Read the model definition and answer for the solid it produces. Units are mm, in the model's axes. Face numbers are marked on the shaded views. Give positions to 0.01 mm unless a question says otherwise; leave off trailing zeros. Order: outer loops, then holes, each group sorted by start corner. A loop starts at its lowest first (then second) coordinate and runs counter-clockwise, first axis right, second up. Notation, with made-up numbers: M -7.75,74.5 L 35.25,74.5 A33 ccw 35.25,106.5 Z; hole C 51.25,34.5 d9. An arc over 180 degrees is marked long. One line per item, written item: value.
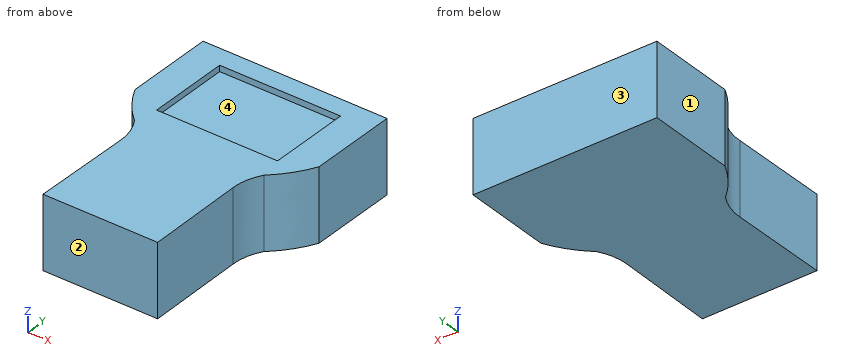
from build123d import *

# Parameters (mm, degrees)
BOSS_EXTRUDE1_DEPTH = 30
SKETCH2_W           = 50.095183997
SKETCH2_H           = 33.986838613
CUT_EXTRUDE1_DEPTH  = 2.5


with BuildPart() as part:
    # Sketch1 → Boss-Extrude1 (new body)
    with BuildSketch(Plane.XY):
        with BuildLine():
            Line((31.309465796, -34.490317077), (31.723853575, -75.590275849))
            Line((31.723853575, -75.590275849), (-15.789641544, -75.590275849))
            Line((-15.789641544, -75.590275849), (-15.375253765, -34.490317077))
            add(Edge.make_bspline(
                [(-18.877545921, -22.198221739), (-16.498314262, -25.992208525), (-15.330883543, -30.089573637), (-15.375253765, -34.490317077)],
                knots=[0, 0, 0, 0, 1, 1, 1, 1], degree=3))
            add(Edge.make_bspline(
                [(-30.14454169, -7.27706518), (-25.994179114, -15.945334243), (-18.877545921, -22.198221739)],
                knots=[0, 0, 0, 1, 1, 1], degree=2))
            Line((-30.14454169, -7.27706518), (-30.14454169, 29.385543018))
            Line((-30.14454169, 29.385543018), (25.046286628, 29.385543018))
            Line((25.046286628, 29.385543018), (46.078753721, 29.385543018))
            Line((46.078753721, 29.385543018), (46.078753721, -7.27706518))
            add(Edge.make_bspline(
                [(46.078753721, -7.27706518), (41.928391145, -15.945334243), (34.811757952, -22.198221739)],
                knots=[0, 0, 0, 1, 1, 1], degree=2))
            add(Edge.make_bspline(
                [(34.811757952, -22.198221739), (32.432526292, -25.992208525), (31.265095574, -30.089573637), (31.309465796, -34.490317077)],
                knots=[0, 0, 0, 0, 1, 1, 1, 1], degree=3))
        make_face()
    extrude(amount=BOSS_EXTRUDE1_DEPTH)

    # Sketch2 → Cut-Extrude1 (cut)
    with BuildSketch(Plane.XY.offset(30)):
        with Locations((8.055613407, 4.246417782)):
            Rectangle(SKETCH2_W, SKETCH2_H)
    extrude(amount=-CUT_EXTRUDE1_DEPTH, mode=Mode.SUBTRACT)


solid = part.part
1) Find section B-B, the plane y = 2. Write down the section's boundary in (x, z).
Reported:
outline: M -30.14,0 L 46.08,0 L 46.08,30 L 33.1,30 L 33.1,27.5 L -16.99,27.5 L -16.99,30 L -30.14,30 Z
2) Find section C-C, the plane y = -41.5. Write down the section's boundary in (x, z), plus the area to 3 significant figures.
Reported:
outline: M -15.45,0 L 31.38,0 L 31.38,30 L -15.45,30 Z
area: 1,400 mm^2
3) Consider probe 1 along X at (y, z) = (-34.5, 20.5); probe 2 along Y at (x, z) = (42, 17); probe 3 along Y at (x, z) = (-22.5, 23). Determine where each line is inside the solid, lowest interval first.
Reported:
probe 1: x = -15.38 to 31.31
probe 2: y = -14.23 to 29.39
probe 3: y = -18.65 to 29.39
4) Determine the mould class of the marked faces 1, 2, 3 and 4 for opening direction Y: +Y half, -Y half, draft (parallel to the pull), parting line (faces both ways), or undercut.
Reported:
face 1: draft
face 2: -Y half
face 3: +Y half
face 4: undercut
5) Each of these flat-tipped pins is pushed along its axis until it touches: pin 1 Ø10 at (y, z) = (-50.5, 14.5) entering from -X; pin 2 Ø10 at (x, y) = (-18, -64) entering from -Z; pin 3 Ø10 at (y, z) = (-29.5, 13.5) entering from +X (3 decimals); pin 4 Ø10 at (x, y) = (10.5, 10) entering from +Z. Where does it stop, or does it pass through?
Reported:
pin 1: stops at x = -15.59
pin 2: stops at z = 0
pin 3: stops at x = 33.535
pin 4: stops at z = 27.5
6) Find section D-D, the plane y = -61. Write down the section's boundary in (x, z).
Reported:
outline: M -15.64,0 L 31.58,0 L 31.58,30 L -15.64,30 Z
7) Find section A-A, the plane x = 16. Write down the section's boundary in (y, z).
Reported:
outline: M -75.59,0 L 29.39,0 L 29.39,30 L 21.24,30 L 21.24,27.5 L -12.75,27.5 L -12.75,30 L -75.59,30 Z
